Check sheet for the drawn part. Datum: minimum x, y, z corner. Units: mm. Give positions to 0.01 mm unless a question says otherwise; leave off trailing zeros. Loops run counter-clockwise (first coordinate to the right, second up) from the corner with the lowest first, then second, coordinate; pieces in that order, holes last. Notation, with made-up numbers: (-22, 77) - (11, 77) arc R17 ccw to (11, 90) - close; hole circle Ø9 at (-37, -30). An arc over 180 degrees is marked (long way). Use one line per item in the form item = value.
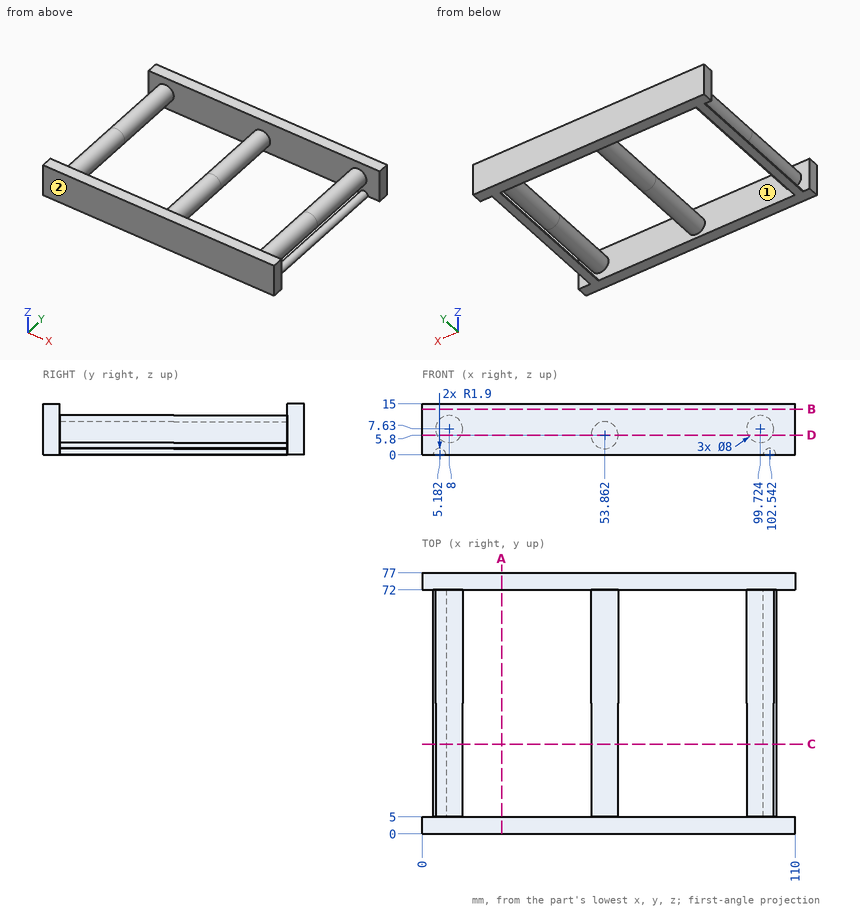
1. Section check C-C, the plane y = 26.5. Record the cut outline in (x, z), then the cut area to 3 significant figures.
Result set:
outline = (3.28, 0) - (7.08, 0) arc R1.9 ccw to start; circle Ø8 at (8, 7.63); circle Ø8 at (53.86, 5.8); circle Ø8 at (99.72, 7.63); (100.64, 0) - (104.44, 0) arc R1.9 ccw to start
area = 162 mm²
2. Depth check by flat-ended pin: pin 1 Ø6 at (y, z) = (46.5, 13) entering from -X; pin 2 Ø2 at (y, z) = (17, 7.5) entering from -X. Enter the tip coordinate at first touch or a pass-through.
Result set:
pin_1 = 4.78
pin_2 = 4
3. Section check D-D, the plane z = 5.8. Record the cut outline in (x, y), then the cut area to 3 significant figures.
Result set:
outline = (0, 0) - (110, 0) - (110, 5) - (103.28, 5) - (103.28, 72) - (110, 72) - (110, 77) - (0, 77) - (0, 72) - (4.44, 72) - (4.44, 5) - (0, 5) - close; hole (11.56, 5) - (49.86, 5) - (49.86, 72) - (11.56, 72) - close; hole (57.86, 5) - (96.17, 5) - (96.17, 72) - (57.86, 72) - close
area = 2,590 mm²
4. Scan lines: probe 1 along Y at (x, z) = (71, 10.75); probe 2 along X at (y, z) = (29.5, 6.25) (1 decimal); probe 3 along X at (y, z) = (58, 7.75) (1 decimal). Record each from-to range of solid material in increasing order.
Result set:
probe_1 = 0 to 5, 72 to 77
probe_2 = 4.2 to 11.8, 49.9 to 57.8, 96 to 103.5
probe_3 = 4 to 12, 50.4 to 57.4, 95.7 to 103.7
5. Draft check along X on the marked faces 1 and 2. Enter one of: released by +X, released by -X, zero draft, split by the parting line, or undercut.
Result set:
face_1 = undercut
face_2 = zero draft
6. Section check B-B, the plane z = 13.5. Record the cut outline in (x, y).
Result set:
outline = (0, 0) - (110, 0) - (110, 5) - (0, 5) - close; (0, 72) - (110, 72) - (110, 77) - (0, 77) - close
7. Section check A-A, the plane x = 23.5. Record the cut outline in (y, z).
Result set:
outline = (0, 0) - (5, 0) - (5, 15) - (0, 15) - close; (72, 0) - (77, 0) - (77, 15) - (72, 15) - close
